For this review, use the dimensioned drawing (mm, ordinates from the lowest corner) and the shaded views. A direction names the side the tool comes from. Round coordinates to 2 decimals unless told otherwise and drop trailing zeros. Write each loop counter-clockwise with the first axis right and the second up, starting at its lowest first coordinate (ties: lowest second). Pieces come first, ordered by that corner, then holes. Notation, with made-up numbers: (-13, 74.5) -> (17, 74.5) arc R19 cw to (17, 83.5) -> close; hole circle Ø4 at (46.5, -20). An arc over 180 degrees is marked (long way). Answer in a Markdown table with one row per item. Add a question column.
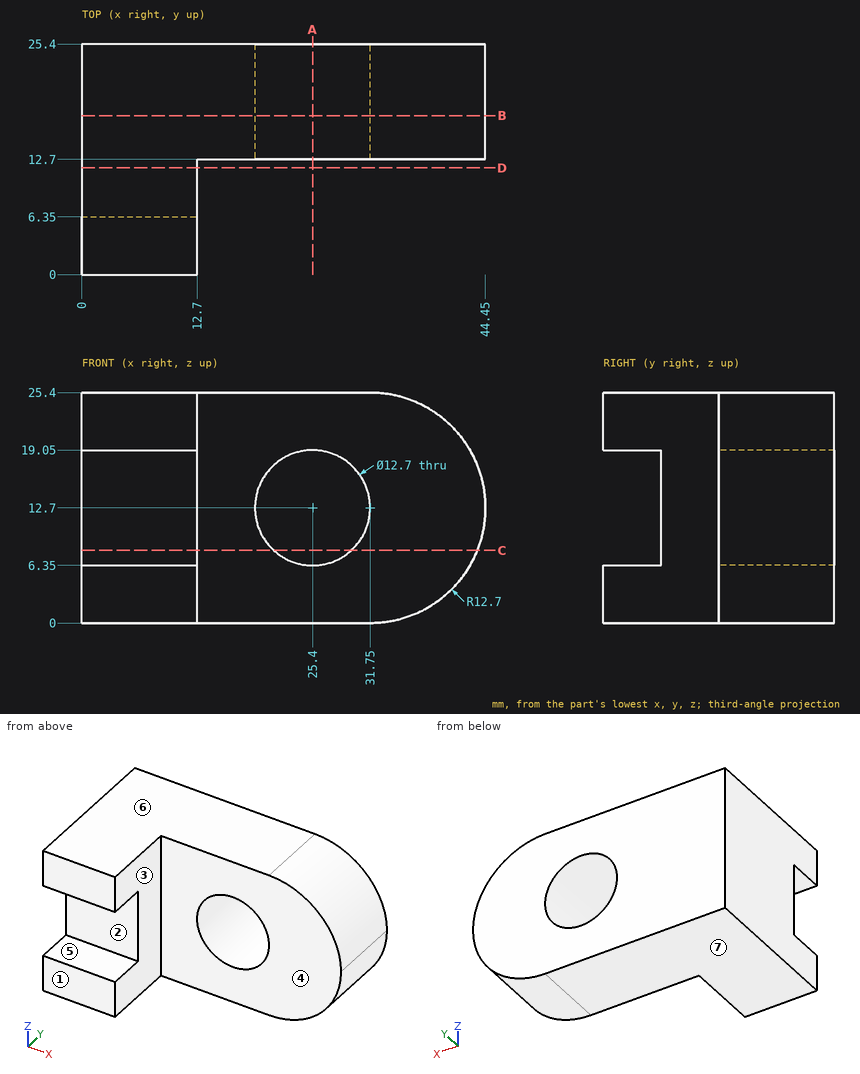
1. Clearance check with flat-ended pins moving along their axes: pin 1 Ø10 at (x, z) = (18, 7) entering from -Y; pin 2 Ø10 at (y, z) = (12.5, 7.5) entering from +X; pin 3 Ø6.5 at (y, z) = (6.5, 11) entering from +X. State where each tip first meets the part, or that it passes through.
2. Tool access review of the marked faces 1, 2 and 3: name each direction out of +Z, -Z, +X, -X, +Y, -Y from which nothing blocks a thin tool from reaching the whole face with its end or side.
3. We need section D-D (y = 11.75). Write out the cut boundary in (x, z), plus the area to 3 significant figures.
4. For L1, parallel to Z at x = 25.4, y = 17.25; L2, parallel to Y at x = 21, z = 5; L3, parallel to X at y = 14, z = 7.75, list the stretches that pass through material, from the lowest coordinate up. Write a range as [from, to].
5. We need section A-A (x = 25.4). Write out the cut boundary in (y, z).
6. We need section C-C (z = 8). Write out the cut boundary in (x, y), plus the area to 3 significant figures.
7. The part is to be moulded in two halves that separate along Z. For the marked faces 4, 5, 6 and 7, say which applies: pulls with the +Z half, pulls with the -Z half, needs draft (parallel to the pull), parting line crosses it, or undercut.
8. We need section B-B (y = 17.5). Write out the cut boundary in (x, z), plus the area to 3 significant figures.
Response:
| question | item | result |
|---|---|---|
| 1 | pin 1 | y = 12.7 |
| 1 | pin 2 | x = 44.45 |
| 1 | pin 3 | x = 12.7 |
| 2 | face 1 | +Z, -Z, +X, -X, -Y |
| 2 | face 2 | +X, -X, -Y |
| 2 | face 3 | +Z, -Z, +X, -Y |
| 3 | outline | (0, 0) -> (12.7, 0) -> (12.7, 25.4) -> (0, 25.4) -> close |
| 3 | area | 323 mm2 |
| 4 | L1 | [0, 6.35], [19.05, 25.4] |
| 4 | L2 | [12.7, 25.4] |
| 4 | L3 | [0, 21.42], [29.38, 43.45] |
| 5 | outline | (12.7, 0) -> (25.4, 0) -> (25.4, 6.35) -> (12.7, 6.35) -> close; (12.7, 19.05) -> (25.4, 19.05) -> (25.4, 25.4) -> (12.7, 25.4) -> close |
| 6 | outline | (0, 6.35) -> (12.7, 6.35) -> (12.7, 12.7) -> (21.13, 12.7) -> (21.13, 25.4) -> (0, 25.4) -> close; (29.67, 12.7) -> (43.55, 12.7) -> (43.55, 25.4) -> (29.67, 25.4) -> close |
| 6 | area | 525 mm2 |
| 7 | face 4 | needs draft |
| 7 | face 5 | undercut |
| 7 | face 6 | pulls with the +Z half |
| 7 | face 7 | pulls with the -Z half |
| 8 | outline | (0, 0) -> (31.75, 0) arc R12.7 ccw to (31.75, 25.4) -> (0, 25.4) -> close; hole circle Ø12.7 at (25.4, 12.7) |
| 8 | area | 933 mm2 |
